from build123d import *

# Parameters (mm, degrees)
SKETCH2_W           = 355.6
SKETCH2_H           = 165.1
SKETCH2_R           = 31.75
SKETCH2_R_2         = 6.35
BOSS_EXTRUDE1_DEPTH = 3.175
CUT_EXTRUDE1_DEPTH  = 4.175
CUT_EXTRUDE3_DEPTH  = 4.175


with BuildPart() as part:
    # Sketch2 → Boss-Extrude1 (new body)
    with BuildSketch(Plane.XY):
        with Locations((95.25, 0)):
            Rectangle(SKETCH2_W, SKETCH2_H)
        Circle(SKETCH2_R, mode=Mode.SUBTRACT)
        with Locations((-54.018973032, 17.551828308)):
            Circle(SKETCH2_R_2, mode=Mode.SUBTRACT)
        with Locations((0, 56.798909535)):
            Circle(SKETCH2_R_2, mode=Mode.SUBTRACT)
        with Locations((54.018973032, 17.551828308)):
            Circle(SKETCH2_R_2, mode=Mode.SUBTRACT)
        with Locations((33.385561371, -45.951283076)):
            Circle(SKETCH2_R_2, mode=Mode.SUBTRACT)
        with Locations((-33.385561371, -45.951283076)):
            Circle(SKETCH2_R_2, mode=Mode.SUBTRACT)
    extrude(amount=BOSS_EXTRUDE1_DEPTH)

    # Sketch3 → Cut-Extrude1 (cut, through all)
    with BuildSketch(Plane.XY.offset(3.175)):
        with BuildLine():
            Line((149.225, -9.525), (130.175, -9.525))
            ThreePointArc((130.175, -9.525), (127, -6.35), (130.175, -3.175))
            Line((130.175, -3.175), (149.225, -3.175))
            ThreePointArc((149.225, -3.175), (152.4, -6.35), (149.225, -9.525))
        make_face()
        with BuildLine():
            Line((250.825, -9.525), (231.775, -9.525))
            ThreePointArc((231.775, -9.525), (228.6, -6.35), (231.775, -3.175))
            Line((231.775, -3.175), (250.825, -3.175))
            ThreePointArc((250.825, -3.175), (254, -6.35), (250.825, -9.525))
        make_face()
        with BuildLine():
            Line((238.125, -60.325), (219.075, -60.325))
            ThreePointArc((219.075, -60.325), (215.9, -57.15), (219.075, -53.975))
            Line((219.075, -53.975), (238.125, -53.975))
            ThreePointArc((238.125, -53.975), (241.3, -57.15), (238.125, -60.325))
        make_face()
        with BuildLine():
            Line((142.875, -53.975), (161.925, -53.975))
            ThreePointArc((161.925, -53.975), (165.1, -57.15), (161.925, -60.325))
            Line((161.925, -60.325), (142.875, -60.325))
            ThreePointArc((142.875, -60.325), (139.7, -57.15), (142.875, -53.975))
        make_face()
    extrude(amount=-CUT_EXTRUDE1_DEPTH, mode=Mode.SUBTRACT)

    # Sketch4 → Cut-Extrude3 (cut, through all)
    with BuildSketch(Plane.XY.offset(3.175)):
        with BuildLine():
            Line((247.65, 28.575), (247.65, 50.8))
            ThreePointArc((247.65, 50.8), (245.790128061, 55.290128061), (241.3, 57.15))
            Line((241.3, 57.15), (112.395, 57.15))
            ThreePointArc((112.395, 57.15), (107.904871939, 55.290128061), (106.045, 50.8))
            Line((106.045, 50.8), (106.045, 28.575))
            ThreePointArc((106.045, 28.575), (107.904871939, 24.084871939), (112.395, 22.225))
            Line((112.395, 22.225), (241.3, 22.225))
            ThreePointArc((241.3, 22.225), (245.790128061, 24.084871939), (247.65, 28.575))
        make_face()
    extrude(amount=-CUT_EXTRUDE3_DEPTH, mode=Mode.SUBTRACT)


solid = part.part
Can you work these out from the model? Positions are in its coordinate system, mm. A direction names the side the tool comes from. Coordinates: 2 decimals unless noted, no trailing zeros. Write each loop counter-clockwise with the first axis right and the second up, starting at its lowest first coordinate (ties: lowest second). Pieces come first, ordered by that corner, then holes. Notation, with made-up numbers: (6, 22.5) -> (24, 22.5) arc R22 ccw to (24, 49.5) -> close; hole circle Ø8 at (48.5, 70). An arc over 180 degrees is marked (long way). Write each question's results on one line, items separated by ' | '. Start each with the question number.
Q1. Imagine slicing it at A-A (x = 0). Write out the boundary of the cut face in (y, z) (3 decimals).
Q2. Imagine slicing it at B-B (y = -57.15). Write out the boundary of the cut face in (x, z) (3 decimals).
Q3. If I drill on probe 1 along Y at (x, z) = (0, 0.75); probe 2 along Y at (x, z) = (137, 0.25) (3 decimals); probe 3 along X at (y, z) = (29.5, 0.25) (3 decimals), over which ranges is the centre line in solid material (lowest first)?
Q4. We'd pull the mould along X, two halves only. Please class faces 3 (the face through (93, 1, 3.175)), 4 (the face through (-0.8, 63.1, 1.6)): +X half, -X half, draft (parallel to the pull), parting line (faces both ways), or undercut.
Q5. On a 3-axis mill with a long thin cutter (end or side, diameter ignored), from which of +Z, -Z, +X, -X, +Y, -Y can I reach the whole of each face in a straight line? I mean faces 1 (the face through (245.84, 55.24, 1.61)), 2 (the face through (93, 1, 0)). Say none if no direction works.
Q6. Imagine slicing it at C-C (x = 175.5). Write out the boundary of the cut face in (y, z) (3 decimals), then the cut area to 3 significant figures.
Q7. Imagine slicing it at D-D (y = 0). Write out the boundary of the cut face in (x, z) (3 decimals).
Taken from the geometry:
1) outline: (-82.55, 0) -> (-31.75, 0) -> (-31.75, 3.175) -> (-82.55, 3.175) -> close; (31.75, 0) -> (50.449, 0) -> (50.449, 3.175) -> (31.75, 3.175) -> close; (63.149, 0) -> (82.55, 0) -> (82.55, 3.175) -> (63.149, 3.175) -> close
2) outline: (-82.55, 0) -> (139.7, 0) -> (139.7, 3.175) -> (-82.55, 3.175) -> close; (165.1, 0) -> (215.9, 0) -> (215.9, 3.175) -> (165.1, 3.175) -> close; (241.3, 0) -> (273.05, 0) -> (273.05, 3.175) -> (241.3, 3.175) -> close
3) probe 1: y = -82.55 to -31.75, 31.75 to 50.45, 63.15 to 82.55 | probe 2: y = -82.55 to -9.525, -3.175 to 22.225, 57.15 to 82.55 | probe 3: x = -82.55 to -11.739, 11.739 to 106.045, 247.65 to 273.05
4) face 3: draft | face 4: undercut
5) face 1: +Z, -Z | face 2: -Z, +X, -X, +Y, -Y
6) outline: (-82.55, 0) -> (22.225, 0) -> (22.225, 3.175) -> (-82.55, 3.175) -> close; (57.15, 0) -> (82.55, 0) -> (82.55, 3.175) -> (57.15, 3.175) -> close | area: 413 mm^2
7) outline: (-82.55, 0) -> (-31.75, 0) -> (-31.75, 3.175) -> (-82.55, 3.175) -> close; (31.75, 0) -> (273.05, 0) -> (273.05, 3.175) -> (31.75, 3.175) -> close
